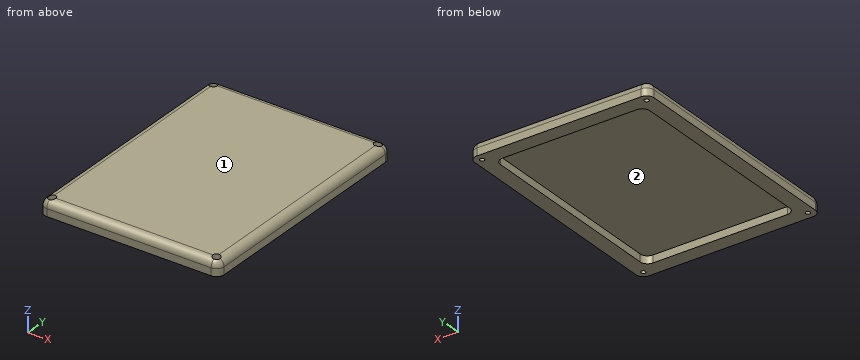
```python
from build123d import *

# Parameters (mm, degrees)
SKETCH1_W           = 120
SKETCH1_H           = 160
BOSS_EXTRUDE1_DEPTH = 10
SKETCH2_W           = 100
SKETCH2_H           = 140
CUT_EXTRUDE1_DEPTH  = 5
FILLET1_R           = 5
FILLET2_R           = 5
FILLET3_R           = 5
SKETCH3_R           = 2.5
CUT_EXTRUDE2_DEPTH  = 5
SKETCH4_R           = 2.5
CUT_EXTRUDE3_DEPTH  = 5
SKETCH5_R           = 2.5
CUT_EXTRUDE4_DEPTH  = 5
SKETCH6_R           = 1.5
CUT_EXTRUDE5_DEPTH  = 10


with BuildPart() as part:
    # Sketch1 → Boss-Extrude1 (new body)
    with BuildSketch(Plane.XY):
        with Locations((60, -80)):
            Rectangle(SKETCH1_W, SKETCH1_H)
    extrude(amount=BOSS_EXTRUDE1_DEPTH)

    # Sketch2 → Cut-Extrude1 (cut)
    with BuildSketch(Plane(origin=(0, 0, 0), x_dir=(-1, 0, 0), z_dir=(0, 0, -1))):
        with Locations((-60, -80)):
            Rectangle(SKETCH2_W, SKETCH2_H)
    extrude(amount=-CUT_EXTRUDE1_DEPTH, mode=Mode.SUBTRACT)

    # Fillet1
    fillet1_edges = [part.edges().sort_by_distance(p)[0] for p in [
        (10, -10, 2.5),
    ]]
    fillet(fillet1_edges, radius=FILLET1_R)

    # Fillet2
    fillet2_edges = [part.edges().sort_by_distance(p)[0] for p in [
        (110, -150, 2.5),
        (110, -10, 2.5),
        (10, -150, 2.5),
    ]]
    fillet(fillet2_edges, radius=FILLET2_R)

    # Fillet3
    fillet3_edges = [part.edges().sort_by_distance(p)[0] for p in [
        (120, -80, 10),
        (60, 0, 10),
        (0, -80, 10),
        (60, -160, 10),
        (0, 0, 5),
        (120, 0, 5),
        (120, -160, 5),
        (0, -160, 5),
    ]]
    fillet(fillet3_edges, radius=FILLET3_R)

    # Sketch3 → Cut-Extrude2 (cut)
    with BuildSketch(Plane.XY.offset(10)):
        with Locations((115, -5)):
            Circle(SKETCH3_R)
    extrude(amount=-CUT_EXTRUDE2_DEPTH, mode=Mode.SUBTRACT)

    # Sketch4 → Cut-Extrude3 (cut)
    with BuildSketch(Plane.XY.offset(10)):
        with Locations((5, -5)):
            Circle(SKETCH4_R)
    extrude(amount=-CUT_EXTRUDE3_DEPTH, mode=Mode.SUBTRACT)

    # Sketch5 → Cut-Extrude4 (cut)
    with BuildSketch(Plane.XY.offset(10)):
        with Locations((5, -155)):
            Circle(SKETCH5_R)
        with Locations((115, -155)):
            Circle(SKETCH5_R)
    extrude(amount=-CUT_EXTRUDE4_DEPTH, mode=Mode.SUBTRACT)

    # Sketch6 → Cut-Extrude5 (cut)
    with BuildSketch(Plane.XY.offset(5)):
        with Locations((5, -5)):
            Circle(SKETCH6_R)
        with Locations((115, -5)):
            Circle(SKETCH6_R)
        with Locations((115, -155)):
            Circle(SKETCH6_R)
        with Locations((5, -155)):
            Circle(SKETCH6_R)
    extrude(amount=-CUT_EXTRUDE5_DEPTH, mode=Mode.SUBTRACT)


solid = part.part
```
Verification items for the finished model (mm, model axes). Face numbers are marked on the shaded views. Coordinates: 2 decimals unless noted, no trailing zeros. Order: outer loops, then holes, each group sorted by start corner. A loop starts at its lowest first (then second) coordinate and runs counter-clockwise, first axis right, second up. Notation, with made-up numbers: (-1.75, 20.5) -> (24.25, 20.5) arc R11 cw to (24.25, 34.5) -> close; hole circle Ø1 at (19.25, 47.5). An arc over 180 degrees is marked (long way). Answer as CSV lines item,"result". Start each with the question number.
1) Cross-section at B-B, the plane y = -74. Record the boundary of the cut face in (x, z), then the cut area to 3 significant figures.
2) Gauge pin test, flat ends, axial feed: pin 1 Ø2.5 at (x, y) = (114, -156) entering from +Z; pin 2 Ø5 at (x, z) = (56, 6) entering from +Y; pin 3 Ø8 at (x, y) = (104.5, -141) entering from -Z; pin 4 Ø4.5 at (x, y) = (5, -155) entering from +Z. Record the tip position at first contact, or that the pin passes through.
3) Release check for a two-part mould opening along X. For the marked faces 1 and 2 record: released by +X, released by -X, zero draft, split by the parting line, or undercut.
4) Material ranges on L1, parallel to X at y = -155, z = 2.75; L2, parallel to Y at x = 5, z = 2.4; L3, parallel to Y at x = 5, z = 8.05, recorded low to high. Write a range as [from, to].
5) Cross-section at A-A, the plane z = 3.25. Record the boundary of the cut face in (x, y), then the cut area to 3 significant figures.
6) Cross-section at C-C, the plane x = 79.5. Record the boundary of the cut face in (y, z).
Conclusion:
1,outline,"(0, 0) -> (10, 0) -> (10, 5) -> (110, 5) -> (110, 0) -> (120, 0) -> (120, 5) arc R5 ccw to (115, 10) -> (5, 10) arc R5 ccw to (0, 5) -> close"
1,area,"689 mm²"
2,pin 1,"stops at z = 9.88"
2,pin 2,"stops at y = 0"
2,pin 3,"stops at z = 5"
2,pin 4,"stops at z = 5"
3,face 1,"zero draft"
3,face 2,"undercut"
4,L1,"x = [0, 3.5], [6.5, 113.5], [116.5, 120]"
4,L2,"y = [-160, -156.5], [-153.5, -6.5], [-3.5, 0]"
4,L3,"y = [-158.96, -157.5], [-152.5, -7.5], [-2.5, -1.04]"
5,outline,"(0, -155) arc R5 ccw to (5, -160) -> (115, -160) arc R5 ccw to (120, -155) -> (120, -5) arc R5 ccw to (115, 0) -> (5, 0) arc R5 ccw to (0, -5) -> close; hole circle Ø3 at (5, -155); hole circle Ø3 at (5, -5); hole (10, -145) arc R5 ccw to (15, -150) -> (105, -150) arc R5 ccw to (110, -145) -> (110, -15) arc R5 ccw to (105, -10) -> (15, -10) arc R5 ccw to (10, -15) -> close; hole circle Ø3 at (115, -155); hole circle Ø3 at (115, -5)"
5,area,"5,170 mm²"
6,outline,"(-160, 0) -> (-150, 0) -> (-150, 5) -> (-10, 5) -> (-10, 0) -> (0, 0) -> (0, 5) arc R5 ccw to (-5, 10) -> (-155, 10) arc R5 ccw to (-160, 5) -> close"
